Design review of the part built by this model. Coordinates are the model's own, in mm. Coordinates: 2 decimals unless noted, no trailing zeros. Loops run counter-clockwise (first coordinate to the right, second up) from the corner with the lowest first, then second, coordinate; pieces in that order, holes last.
Autodesk Inventor part; units mm, degrees
ref_plane "YZ Plane" through (0, 0, 0) normal (1, 0, 0) x (0, 1, 0)
ref_plane "XZ Plane" through (0, 0, 0) normal (0, 1, 0) x (-1, 0, 0)
ref_plane "XY Plane" through (0, 0, 0) normal (0, 0, 1) x (1, 0, 0)
sketch "Sketch1" plane through (0, 0, 0) normal (1, 0, 0) x (0, 1, 0)
  line L0 (3.2531, 52.0584) -> (0.3531, 52.0584)
  line L1 (0.3531, 52.0584) -> (0.3531, -10.0416)
  line L2 (0.3531, -10.0416) -> (3.2531, -10.0416)
  line L3 (3.2531, -10.0416) -> (3.2531, 52.0584)
  arc A0 (3.2531, 52.0584) -> (2.9699, 57.9259) centre (1.8031, 54.929) ccw
  arc A1 (0.7699, 57.9745) -> (0.3531, 52.0584) centre (1.8031, 54.929) ccw
  line L4 (0.7699, 57.9745) -> (0.7699, 56.8745)
  line L5 (2.9699, 57.9259) -> (2.9699, 56.8259)
  arc A2 (0.7699, 56.8745) -> (2.9699, 56.8259) centre (1.8253, 54.832) ccw
  point P0 (0, 0)
  dimension "d0" = 2.9
  dimension "d1" = 62.1
  dimension "d156" = 1.1
  dimension "d157" = 1.1
  dimension "d158" = 2.2
extrude "Extrusion1" add sketch "Sketch1" against normal blind 20
sketch "Sketch3" plane through (0, 0, 0) normal (1, 0, 0) x (0, 0, -1)
  arc A0 (-52.0584, 3.2531) -> (-57.9259, 2.9699) centre (-54.929, 1.8031) ccw
  line L0 (10.0416, 0.3531) -> (-52.0584, 0.3531)
  line L1 (-52.0584, 3.2531) -> (10.0416, 3.2531)
  line L2 (10.0416, 3.2531) -> (10.0416, 0.3531)
  line L3 (10.0416, 0.3531) -> (-52.0584, 0.3531)
  line L4 (-52.0584, 0.3531) -> (-52.0584, 3.2531)
  point P0 (0, 0)
extrude "Extrusion2" add sketch "Sketch3" along normal blind 40
sketch "Sketch4" plane through (40, 0, 0) normal (1, 0, 0) x (0, 0, -1)
  line L0 (10.0416, 0.3531) -> (-52.0584, 0.3531)
  line L1 (10.0416, 0.3531) -> (-52.0584, 0.3531)
  line L2 (-52.0584, 0.3531) -> (-52.0584, 3.2531)
  line L3 (-52.0584, 3.2531) -> (10.0416, 3.2531)
  line L4 (10.0416, 3.2531) -> (10.0416, 0.3531)
  arc A0 (-57.9745, 0.7699) -> (-52.0584, 0.3531) centre (-54.929, 1.8031) ccw
  arc A1 (-57.9745, 0.7699) -> (-52.0584, 0.3531) centre (-54.929, 1.8031) ccw
  arc A2 (-52.0584, 3.2531) -> (-57.9259, 2.9699) centre (-54.929, 1.8031) ccw
  arc A3 (-52.0584, 3.2531) -> (-57.9259, 2.9699) centre (-54.929, 1.8031) ccw
  arc A4 (-56.8745, 0.7699) -> (-56.8259, 2.9699) centre (-54.832, 1.8253) ccw
  arc A5 (-56.8745, 0.7699) -> (-56.8259, 2.9699) centre (-54.832, 1.8253) ccw
  line L5 (-56.8745, 0.7699) -> (-57.9745, 0.7699)
  line L6 (-56.8745, 0.7699) -> (-57.9745, 0.7699)
  line L7 (-57.9259, 2.9699) -> (-56.8259, 2.9699)
  line L8 (-56.8259, 2.9699) -> (-57.9259, 2.9699)
  point P0 (0, 0)
  dimension "d159" = 1.1
  dimension "d160" = 2.2
extrude "Extrusion3" add sketch "Sketch4" along normal blind 20
sketch "Sketch9" plane through (0, 0.3531, 52.0584) normal (0, 0, 1) x (1, 0, 0)
  line L0 (0, 2.9) -> (40, 2.9)
  line L1 (0, 2.9) -> (40, 2.9)
  line L2 (40, 2.9) -> (40, 0)
  line L3 (40, 0) -> (0, 0)
  line L4 (0, 0) -> (0, 2.9)
  point P0 (0, -0.3531)
extrude "Extrusion4" add sketch "Sketch9" along normal blind 6
sketch "Sketch10" plane through (-20, 0, 0) normal (-1, 0, 0) x (0, 0, 1)
  arc A0 (52.0584, 0.3531) -> (57.9745, 0.7699) centre (54.929, 1.8031) ccw
  line L0 (-10.0416, 3.2531) -> (-10.0416, 0.3531)
  line L1 (52.0584, 0.3531) -> (-10.0416, 0.3531)
  line L2 (-10.0416, 0.3531) -> (-10.0416, 3.2531)
  line L3 (-10.0416, 3.2531) -> (52.0584, 3.2531)
  line L4 (52.0584, 3.2531) -> (52.0584, 0.3531)
  point P0 (0, 0)
extrude "Extrusion5" add sketch "Sketch10" along normal blind 10
sketch "Sketch11" plane through (60, 0, 0) normal (1, 0, 0) x (0, 0, -1)
  line L0 (10.0416, 0.3531) -> (10.0416, 3.2531)
  arc A0 (-52.0584, 3.2531) -> (-57.7996, 3.2531) centre (-54.929, 1.8031) ccw
  line L1 (10.0416, 0.3531) -> (-52.0584, 0.3531)
  line L2 (-52.0584, 0.3531) -> (-52.0584, 3.2531)
  line L3 (-52.0584, 3.2531) -> (10.0416, 3.2531)
  line L4 (10.0416, 3.2531) -> (10.0416, 0.3531)
  point P0 (0, 0)
extrude "Extrusion6" add sketch "Sketch11" along normal blind 10
sketch "Sketch5" plane through (-20, 0.3531, -10.0416) normal (0, -1, 0) x (1, 0, 0)
  line L0 (20, 62.1) -> (60, 62.1)
  line L1 (0, 0) -> (0, 62.1)
  line L2 (60, 68.1) -> (20, 68.1)
  line L3 (-10, 0) -> (-10, 62.1)
  point P0 (20, 10.0416)
  point P1 (30.525, 64.15)
  dimension "d80" = 40.525
  dimension "d81" = 3.95
hole "Hole1" at (10.525, 0.3531, 54.1084) direction (0, 1, 0) diameter 2.921 end through all
sketch "Sketch6" plane through (-20, 0.3531, -10.0416) normal (0, -1, 0) x (1, 0, 0)
  line L0 (20, 62.1) -> (60, 62.1)
  circle A0 centre (30.525, 64.15) radius 1.4605
  line L1 (60, 68.1) -> (20, 68.1)
  point P0 (20, 10.0416)
  point P1 (49.475, 64.15)
  dimension "d42" = 18.95
  dimension "d53" = 3.95
hole "Hole2" at (29.475, 0.3531, 54.1084) direction (0, 1, 0) diameter 2.921 end through all
sketch "Sketch7" plane through (-20, 0.3531, -10.0416) normal (0, -1, 0) x (1, 0, 0)
  line L0 (0, 0) -> (0, 62.1)
  circle A0 centre (30.525, 64.15) radius 1.4605
  line L1 (-10, 0) -> (-10, 62.1)
  point P0 (20, 10.0416)
  point P1 (30.525, 2.76)
  dimension "d49" = 61.39
  dimension "d82" = 40.525
hole "Hole3" at (10.525, 0.3531, -7.2816) direction (0, 1, 0) diameter 2.921 end through all
sketch "Sketch8" plane through (-20, 0.3531, -10.0416) normal (0, -1, 0) x (1, 0, 0)
  circle A0 centre (30.525, 2.76) radius 1.4605
  circle A1 centre (49.475, 64.15) radius 1.4605
  point P0 (20, 10.0416)
  point P1 (49.475, 2.76)
  point P2 (41.1972, 0)
  point P3 (38.7028, 0)
  point P4 (60, 64.989)
  point P5 (60, 63.311)
  dimension "d48" = 18.95
  dimension "d54" = 61.39
hole "Hole4" at (29.475, 0.3531, -7.2816) direction (0, 1, 0) diameter 2.921 end through all
sketch "Sketch12" plane through (0, 0.3531, 58.0584) normal (0, -1, 0) x (1, 0, 0)
  line L0 (-20, -6) -> (-30, -6)
  line L1 (-30, -68.1) -> (-30, -6)
  point P0 (0, -58.0584)
  point P1 (-24.59, -14.57)
  dimension "d133" = 8.57
  dimension "d134" = 5.41
hole "Hole5" at (-24.59, 0.3531, 43.4884) direction (0, 1, 0) diameter 2.921 end through all
sketch "Sketch13" plane through (0, 0.3531, 58.0584) normal (0, -1, 0) x (1, 0, 0)
  line L0 (0, -6) -> (-20, -6)
  circle A0 centre (-24.59, -14.57) radius 1.4605
  point P0 (0, -58.0584)
  point P1 (-11.33, -14.57)
  dimension "d135" = 8.57
  dimension "d136" = 13.26
hole "Hole6" at (-11.33, 0.3531, 43.4884) direction (0, 1, 0) diameter 2.921 end through all
sketch "Sketch14" plane through (0, 0.3531, 58.0584) normal (0, -1, 0) x (1, 0, 0)
  line L0 (-30, -68.1) -> (-30, -6)
  circle A0 centre (-24.59, -14.57) radius 1.4605
  point P0 (0, -58.0584)
  point P1 (-24.59, -59.53)
  dimension "d137" = 5.41
  dimension "d138" = 44.96
hole "Hole7" at (-24.59, 0.3531, -1.4716) direction (0, 1, 0) diameter 2.921 end through all
sketch "Sketch15" plane through (0, 0.3531, 58.0584) normal (0, -1, 0) x (1, 0, 0)
  circle A0 centre (-11.33, -14.57) radius 1.4605
  circle A1 centre (-24.59, -59.53) radius 1.4605
  point P0 (0, -58.0584)
  point P1 (-11.33, -59.53)
  dimension "d139" = 44.96
  dimension "d148" = 13.26
hole "Hole8" at (-11.33, 0.3531, -1.4716) direction (0, 1, 0) diameter 2.921 end through all
sketch "Sketch17" plane through (0, 0.3531, 58.0584) normal (0, -1, 0) x (1, 0, 0)
  line L0 (70, -6) -> (70, -68.1)
  line L1 (60, -6) -> (70, -6)
  point P0 (0, -58.0584)
  point P1 (64.59, -14.57)
  dimension "d142" = 5.41
  dimension "d147" = 8.57
hole "Hole10" at (64.59, 0.3531, 43.4884) direction (0, 1, 0) diameter 2.921 end through all
sketch "Sketch16" plane through (0, 0.3531, 58.0584) normal (0, -1, 0) x (1, 0, 0)
  circle A0 centre (64.59, -14.57) radius 1.4605
  line L0 (40, -6) -> (60, -6)
  point P0 (0, -58.0584)
  point P1 (51.33, -14.57)
  dimension "d144" = 13.26
  dimension "d146" = 8.57
hole "Hole9" at (51.33, 0.3531, 43.4884) direction (0, 1, 0) diameter 2.921 end through all
sketch "Sketch19" plane through (0, 0.3531, 58.0584) normal (0, -1, 0) x (1, 0, 0)
  circle A0 centre (64.59, -14.57) radius 1.4605
  line L0 (70, -6) -> (70, -68.1)
  point P0 (0, -58.0584)
  point P1 (64.59, -59.53)
  dimension "d141" = 44.96
  dimension "d143" = 5.41
hole "Hole12" at (64.59, 0.3531, -1.4716) direction (0, 1, 0) diameter 2.921 end through all
sketch "Sketch18" plane through (0, 0.3531, 58.0584) normal (0, -1, 0) x (1, 0, 0)
  circle A0 centre (51.33, -14.57) radius 1.4605
  circle A1 centre (64.59, -59.53) radius 1.4605
  point P0 (0, -58.0584)
  point P1 (51.33, -59.53)
  dimension "d140" = 44.96
  dimension "d145" = 13.26
hole "Hole11" at (51.33, 0.3531, -1.4716) direction (0, 1, 0) diameter 2.921 end through all
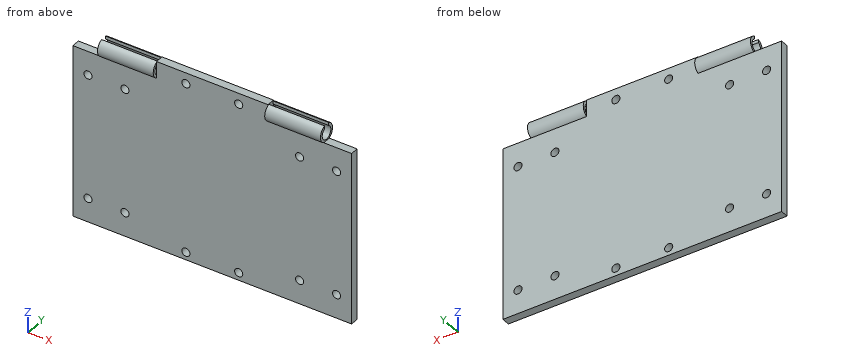
Q1. Take a section at D-D, the plane z = 13. Write out the cut boundary in (x, y).
Q2. For line 1 (Z direction, x = 52, y = 1.5); line 2 (Z direction, x = 64.59, y = 2.05); line 3 (Y direction, x = -19.5, z = 33.5), list the stretches that pass through material, from the lowest coordinate up.
Q3. Clearance check with flat-ended pins moving along their axes: pin 1 Ø8 at (x, z) = (7, 41) entering from -Y; pin 2 Ø1.9 at (y, z) = (-0.5, 54.5) entering from +X; pin 3 Ø1 at (x, z) = (-14.5, 28.5) entering from +Y. State where each tip first meets the part, or that it passes through.
Q4. Take a section at B-B, the plane z = 43.5. Write out the cut boundary in (x, y), then the cut area to 3 significant figures.
Q5. Take a section at C-C, the plane x = 64.59. Write out the cut boundary in (y, z).
Q6. Take a section at A-A, the plane x = -11.33. Write out the cut boundary in (y, z).
Entries:
1. outline: (-30, 0.35) - (70, 0.35) - (70, 3.25) - (-30, 3.25) - close
2. line 1: z = -10.04 to -2.77, -0.17 to 42.19, 44.79 to 52.56
2. line 2: z = -10.04 to -2.93, -0.01 to 42.03, 44.95 to 52.06
2. line 3: y = 0.35 to 3.25
3. pin 1: stops at y = 0.35
3. pin 2: stops at x = 60
3. pin 3: stops at y = 3.25
4. outline: (-30, 0.35) - (-26.05, 0.35) - (-26.05, 3.25) - (-30, 3.25) - close; (-23.13, 0.35) - (-12.79, 0.35) - (-12.79, 3.25) - (-23.13, 3.25) - close; (-9.87, 0.35) - (49.87, 0.35) - (49.87, 3.25) - (-9.87, 3.25) - close; (52.79, 0.35) - (63.13, 0.35) - (63.13, 3.25) - (52.79, 3.25) - close; (66.05, 0.35) - (70, 0.35) - (70, 3.25) - (66.05, 3.25) - close
4. area: 256 mm2
5. outline: (0.35, -10.04) - (3.25, -10.04) - (3.25, -2.93) - (0.35, -2.93) - close; (0.35, -0.01) - (3.25, -0.01) - (3.25, 42.03) - (0.35, 42.03) - close; (0.35, 44.95) - (3.25, 44.95) - (3.25, 52.06) - (0.35, 52.06) - close
6. outline: (0.35, -10.04) - (3.25, -10.04) - (3.25, -2.93) - (0.35, -2.93) - close; (0.35, -0.01) - (3.25, -0.01) - (3.25, 42.03) - (0.35, 42.03) - close; (0.35, 44.95) - (3.25, 44.95) - (3.25, 52.06) arc R3.22 ccw to (2.97, 57.93) - (2.97, 56.83) arc R2.3 cw (long way) to (0.77, 56.87) - (0.77, 57.97) arc R3.22 ccw to (0.35, 52.06) - close
